from build123d import *

# Parameters (mm, degrees)
SKETCH1_R           = 355.6
SKETCH1_R_2         = 279.4
BOSS_EXTRUDE2_DEPTH = 228.6
SKETCH2_R           = 431.8
BOSS_EXTRUDE3_DEPTH = 139.7
SKETCH3_R           = 63.5
BOSS_EXTRUDE4_DEPTH = 76.2
CUT_EXTRUDE1_REACH  = 1159.931
SKETCH4_R           = 279.4


with BuildPart() as part:
    # Sketch1 → Boss-Extrude2 (new body)
    with BuildSketch(Plane(origin=(0, 0, 0), x_dir=(1, 0, 0), z_dir=(0, 1, 0))):
        with Locations(Location((0, 0, 0), (0, 0, 270))):
            Circle(SKETCH1_R)
        with Locations(Location((0, 0, 0), (0, 0, 270))):
            Circle(SKETCH1_R_2, mode=Mode.SUBTRACT)
    extrude(amount=BOSS_EXTRUDE2_DEPTH)

    # Sketch2 → Boss-Extrude3 (add)
    with BuildSketch(Plane(origin=(0, 0, 0), x_dir=(1, 0, 0), z_dir=(0, 1, 0))):
        with Locations(Location((0, 0, 0), (0, 0, 270))):
            Circle(SKETCH2_R)
    extrude(amount=BOSS_EXTRUDE3_DEPTH)

    # Sketch3 → Boss-Extrude4 (add)
    with BuildSketch(Plane(origin=(0, 0, 0), x_dir=(1, 0, 0), z_dir=(0, 1, 0))):
        with BuildLine():
            ThreePointArc((-142.126171723, -715.408284024), (0, -812.8), (142.126171723, -715.408284024))
            ThreePointArc((142.126171723, -715.408284024), (181.782810221, -654.296173404), (242.619424457, -614.218181818))
            ThreePointArc((242.619424457, -614.218181818), (466.973318296, -466.973318296), (614.218181818, -242.619424457))
            ThreePointArc((614.218181818, -242.619424457), (654.296173404, -181.782810221), (715.408284024, -142.126171723))
            ThreePointArc((715.408284024, -142.126171723), (812.8, 0), (715.408284024, 142.126171723))
            ThreePointArc((715.408284024, 142.126171723), (654.296173404, 181.782810221), (614.218181818, 242.619424457))
            ThreePointArc((614.218181818, 242.619424457), (466.973318296, 466.973318296), (242.619424457, 614.218181818))
            ThreePointArc((242.619424457, 614.218181818), (181.782810221, 654.296173404), (142.126171723, 715.408284024))
            ThreePointArc((142.126171723, 715.408284024), (0, 812.8), (-142.126171723, 715.408284024))
            ThreePointArc((-142.126171723, 715.408284024), (-181.782810221, 654.296173404), (-242.619424457, 614.218181818))
            ThreePointArc((-242.619424457, 614.218181818), (-466.973318296, 466.973318296), (-614.218181818, 242.619424457))
            ThreePointArc((-614.218181818, 242.619424457), (-654.296173404, 181.782810221), (-715.408284024, 142.126171723))
            ThreePointArc((-715.408284024, 142.126171723), (-812.8, 0), (-715.408284024, -142.126171723))
            ThreePointArc((-715.408284024, -142.126171723), (-654.296173404, -181.782810221), (-614.218181818, -242.619424457))
            ThreePointArc((-614.218181818, -242.619424457), (-466.973318296, -466.973318296), (-242.619424457, -614.218181818))
            ThreePointArc((-242.619424457, -614.218181818), (-181.782810221, -654.296173404), (-142.126171723, -715.408284024))
        make_face()
        with Locations(Location((0, 660.4, 0), (0, 0, 90))):
            Circle(SKETCH3_R, mode=Mode.SUBTRACT)
        with Locations(Location((660.4, 0, 0), (0, 0, 90))):
            Circle(SKETCH3_R, mode=Mode.SUBTRACT)
        with Locations(Location((0, -660.4, 0), (0, 0, 90))):
            Circle(SKETCH3_R, mode=Mode.SUBTRACT)
        with Locations(Location((-660.4, 0, 0), (0, 0, 90))):
            Circle(SKETCH3_R, mode=Mode.SUBTRACT)
    extrude(amount=BOSS_EXTRUDE4_DEPTH)

    # Sketch4 → Cut-Extrude1 (cut, up to next)
    with BuildSketch(Plane(origin=(0, 139.7, 0), x_dir=(1, 0, 0), z_dir=(0, 1, 0)), mode=Mode.PRIVATE) as cut_extrude1_sk1:
        with Locations(Location((0, 0, 0), (0, 0, 270))):
            Circle(SKETCH4_R)
    cut_extrude1_tool1 = extrude(cut_extrude1_sk1.sketch, amount=-CUT_EXTRUDE1_REACH, mode=Mode.PRIVATE) & part.part
    add(cut_extrude1_tool1.solids().sort_by_distance((0, 139.7, 0))[0], mode=Mode.SUBTRACT)


solid = part.part
Source: CAD feature listing. Evaluate the final solid. Frame: model axes, mm. A direction names the side the tool comes from. Coordinates: 2 decimals unless noted, no trailing zeros. Order: outer loops, then holes, each group sorted by start corner. A loop starts at its lowest first (then second) coordinate and runs counter-clockwise, first axis right, second up. Notation, with made-up numbers: M 76.5,-14.75 L 123.5,-14.75 A27 cw 123.5,22.25 Z; hole C -9.5,-8.5 d6. An arc over 180 degrees is marked long. Write each question's results on one line, items separated by ' | '. Start each with the question number.
1. Reachability of faces 4 (the face through (-2.56, 37.57, 812.78)), 5 (the face through (299.84, 183.53, 191.17)) from +Z, -Z, +X, -X, +Y, -Y: full face, straight path, thin tool, end or side. Return the list, or none.
2. Pin query (flat end, axial travel): pin 1 (8 mm diameter, centred on y = 174.5, z = -37, fed in from -X); pin 2 (12 mm diameter, centred on y = 85, z = -329.5, fed in from -X); pin 3 (2 mm diameter, centred on x = 239.5, y = 130.5, fed in from -Z). Return the tip coordinate at first contact, or that it passes through.
3. Section C-C, the plane x = 660.4. Return the cut outline in (y, z), then the cut area to 3 significant figures.
4. Section A-A, the plane z = 0. Return the cut outline in (x, y), then the cut area to 3 significant figures.
5. Section B-B, the plane y = 52.5. Return the cut outline in (x, z).
6. Draft query along Z for faces 1 (the face through (469.64, 37.57, -464.29)), 2 (the face through (-11, 0, 350)), 3 (the face through (-604.065, 37.567, -29.301)). Return one class per face: +Z half, -Z half, draft (parallel to the pull), parting line (faces both ways), or undercut.
7. Section D-D, the plane y = 198. Return the cut outline in (x, z).
8. Material intervals for L1, parallel to X at y = 58, z = 0; L2, parallel to Z at x = -4, y = 18.5; L3, parallel to X at y = 54, z = -23.5, sorted ascending.
Solution:
1) face 4: +Z, +Y, -Y | face 5: +Y
2) pin 1: x = -354.07 | pin 2: x = -286.01 | pin 3: z = -359.96
3) outline: M 0,-176 L 76.2,-176 L 76.2,-63.5 L 0,-63.5 Z; M 0,63.5 L 76.2,63.5 L 76.2,176 L 0,176 Z | area: 17,100 mm²
4) outline: M -812.8,0 L -723.9,0 L -723.9,76.2 L -812.8,76.2 Z; M -596.9,0 L -279.4,0 L -279.4,228.6 L -355.6,228.6 L -355.6,139.7 L -431.8,139.7 L -431.8,76.2 L -596.9,76.2 Z; M 279.4,0 L 596.9,0 L 596.9,76.2 L 431.8,76.2 L 431.8,139.7 L 355.6,139.7 L 355.6,228.6 L 279.4,228.6 Z; M 723.9,0 L 812.8,0 L 812.8,76.2 L 723.9,76.2 Z | area: 94,800 mm²
5) outline: M -715.41,-142.13 A177.8 cw -614.22,-242.62 A660.4 ccw -242.62,-614.22 A177.8 cw -142.13,-715.41 A152.4 ccw 142.13,-715.41 A177.8 cw 242.62,-614.22 A660.4 ccw 614.22,-242.62 A177.8 cw 715.41,-142.13 A152.4 ccw 715.41,142.13 A177.8 cw 614.22,242.62 A660.4 ccw 242.62,614.22 A177.8 cw 142.13,715.41 A152.4 ccw -142.13,715.41 A177.8 cw -242.62,614.22 A660.4 ccw -614.22,242.62 A177.8 cw -715.41,142.13 A152.4 ccw Z; hole C -660.4,0 d127; hole C 0,0 d558.8; hole C 0,-660.4 d127; hole C 0,660.4 d127; hole C 660.4,0 d127
6) face 1: -Z half | face 2: draft | face 3: undercut
7) outline: C 0,0 d711.2; hole C 0,0 d558.8
8) L1: -812.8 to -723.9, -596.9 to -279.4, 279.4 to 596.9, 723.9 to 812.8 | L2: -812.75 to -723.77, -597.03 to -279.37, 279.37 to 597.03, 723.77 to 812.75 | L3: -810.98 to -719.39, -601.41 to -278.41, 278.41 to 601.41, 719.39 to 810.98
